Autodesk Inventor part; units mm, degrees
ref_plane "YZ Plane" through (0, 0, 0) normal (1, 0, 0) x (0, 1, 0)
ref_plane "XZ Plane" through (0, 0, 0) normal (0, 1, 0) x (-1, 0, 0)
ref_plane "XY Plane" through (0, 0, 0) normal (0, 0, 1) x (1, 0, 0)
sketch "Sketch1" plane through (0, 0, 0) normal (0, 1, 0) x (-1, 0, 0)
  circle A0 centre (0, 0) radius 3.375
  line L0 (0, -3.375) -> (0, 13.925)
  circle A1 centre (0, 11.925) radius 2
  line L1 (1.9867, 12.1556) -> (3.3525, 0.3892)
  line L2 (-1.9867, 12.1556) -> (-3.3525, 0.3892)
  dimension "d0" = 6.75
  dimension "d1" = 17.3
  dimension "d2" = 4
extrude "Extrusion1" add sketch "Sketch1" along normal blind 1.75
sketch "Sketch2" plane through (0, 1.75, 0) normal (0, 1, 0) x (1, 0, 0)
  arc A0 (3.3525, -0.3892) -> (-3.3525, -0.3892) centre (0, 0) ccw
  line L0 (-3.3525, -0.3892) -> (-1.9867, -12.1556)
  arc A1 (-3.3525, -0.3892) -> (3.3525, -0.3892) centre (0, 0) ccw
  circle A2 centre (0, 0) radius 2.875
  dimension "d5" = 5.75
extrude "Extrusion2" add sketch "Sketch2" along normal blind 2.55
sketch "Sketch3" plane through (0, 0, 0) normal (0, -1, 0) x (1, 0, 0)
  arc A0 (-3.3525, 0.3892) -> (3.3525, 0.3892) centre (0, 0) ccw
  circle A1 centre (0, 0) radius 2.375
  dimension "d8" = 4.75
extrude "Extrusion3" cut sketch "Sketch3" against normal blind 1
sketch "Sketch4" plane through (0, 1, 0) normal (0, -1, 0) x (1, 0, 0)
  circle A0 centre (0, 0) radius 1.25
  dimension "d11" = 2.5
extrude "Extrusion4" cut sketch "Sketch4" against normal up to next
sketch "Sketch5" plane through (0, 1.75, 0) normal (0, 1, 0) x (1, 0, 0)
  arc A0 (-1.9867, -12.1556) -> (1.9867, -12.1556) centre (0, -11.925) ccw
  arc A1 (-3.3525, -0.3892) -> (3.3525, -0.3892) centre (0, 0) ccw
  line L0 (0, -3.375) -> (0, -5.1333)
  line L1 (0, -5.1333) -> (0, -6.8917)
  line L2 (0, -6.8917) -> (0, -8.65)
  line L3 (0, -8.65) -> (0, -10.4083)
  line L4 (0, -10.4083) -> (0, -12.1667)
  line L5 (0, -12.1667) -> (0, -13.925)
hole "Hole1" at (0, 1.75, 5.1333) at (0, 1.75, 6.8917) at (0, 1.75, 8.65) at (0, 1.75, 10.4083) at (0, 1.75, 12.1667) direction (0, -1, 0) diameter 1 end through all
properties part number "Small Continuous Servo Horn"
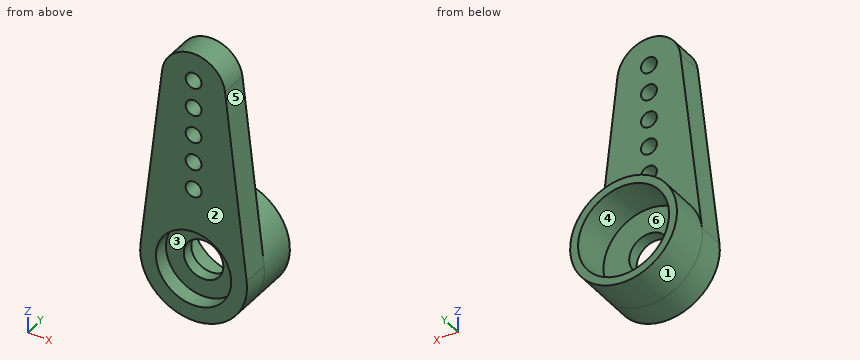
Can you work these out from the model? Positions are in its coordinate system, mm. Face numbers are marked on the shaded views. A direction names the side the tool comes from. Round coordinates to 2 decimals unless told otherwise and drop trailing zeros. Order: outer loops, then holes, each group sorted by start corner. A loop starts at its lowest first (then second) coordinate and runs counter-clockwise, first axis right, second up. Notation, with made-up numbers: (63, -26) -> (114, -26) arc R30 ccw to (114, 9) -> close; hole circle Ø11 at (-22.75, 83.25). An arc over 180 degrees is marked (long way). Return JSON: item names as keys, results as strings. Group by question number.
1. If we section it at B-B, the plane x = 0: Count the separate pieces of the cut face and the enclosed holes in it, then the cut area to 3 significant figures.
2. If we section it at A-A, the plane z = 0: Write out the boundary of the cut face in (x, y) (3 decimals), then the cut area to 3 significant figures.
3. If we section it at C-C, the plane x = -1: Write out the boundary of the cut face in (y, z).
4. We'd pull the mould along Z, two halves only. Please class the marked faces 1, 2, 3 and 4: released by +Z, released by -Z, zero draft, split by the parting line, or undercut.
5. I need wall thicknesses on line 1 (Y direction, x = 1, z = 7); line 2 (Z direction, x = 0, y = 3) (3 decimals); line 3 (Z direction, x = -1, y = 0.2). Which ranges of each line are inside material? Lowest first, please. Write a range as [from, to].
6. Which directions (+Z, -Z, +X, -X, +Y, -Y) give clear straight access to the entire face, cutting with the end or side of a thin tool? Please do the marked faces 5 and 6.
7. Will these pins go through, and if not, where does the flat tip stop? pin 1 (2 mm diameter, centred on y = 1, z = 1.5, fed in from -X); pin 2 (2 mm diameter, centred on x = 0, z = 0, fed in from -Y); pin 3 (3 mm diameter, centred on x = -0.5, z = 0.5, fed in from +Y); pin 4 (1.4 mm diameter, centred on x = 0.5, z = -0.5, fed in from -Y).
Output values:
{
 "1": {"separate pieces": "7", "enclosed holes": "0", "area": "17.5 mm²"},
 "2": {"outline": "(-3.375, 0) -> (-2.375, 0) -> (-2.375, 1) -> (-1.25, 1) -> (-1.25, 1.75) -> (-2.875, 1.75) -> (-2.875, 4.3) -> (-3.375, 4.3) -> close; (1.25, 1) -> (2.375, 1) -> (2.375, 0) -> (3.375, 0) -> (3.375, 4.3) -> (2.875, 4.3) -> (2.875, 1.75) -> (1.25, 1.75) -> close", "area": "7.74 mm²"},
 "3": {"outline": "(0, -3.22) -> (4.3, -3.22) -> (4.3, -2.7) -> (1.75, -2.7) -> (1.75, -0.75) -> (1, -0.75) -> (1, -2.15) -> (0, -2.15) -> close; (0, 2.15) -> (1, 2.15) -> (1, 0.75) -> (1.75, 0.75) -> (1.75, 2.7) -> (4.3, 2.7) -> (4.3, 3.22) -> (1.75, 3.22) -> (1.75, 13.66) -> (0, 13.66) -> close"},
 "4": {"face 1": "split by the parting line", "face 2": "zero draft", "face 3": "undercut", "face 4": "undercut"},
 "5": {"line 1": "[0, 1.75]", "line 2": "[-3.375, -2.875], [2.875, 3.375]", "line 3": "[-3.22, -2.15], [2.15, 13.66]"},
 "6": {"face 5": "+Z, +X, +Y, -Y", "face 6": "+Y"},
 "7": {"pin 1": "x = -3.34", "pin 2": "through", "pin 3": "y = 1.75", "pin 4": "y = 1"}
}
